Input: part model. Units: mm. Frame: model coordinates. A direction names the side the tool comes from. Round coordinates to 2 decimals unless told otherwise and drop trailing zeros. Loops run counter-clockwise (first coordinate to the right, second up) from the corner with the lowest first, then second, coordinate; pieces in that order, holes last.
(1) Access query for faces 5 (the face through (-0.8, -9.6, 200)), 6 (the face through (-0.521, 9.507, -138.034)), 7 (the face through (9, 0, 3)). Directions: +Z, -Z, +X, -X, +Y, -Y. A direction counts if a zero-diameter tool reaches every point of the face in a straight line with its end or side. Return the directions, or none.
(2) Cut plane A-A, the plane z = -79. Output: boundary loops of the cut face in (x, y).
(3) Line query: line 1 (Y direction, x = 7, z = -19); line 2 (X direction, y = 9.75, z = 189.5) (3 decimals). Output: solid intervals per line, ascending.
(4) Draft query along Z for faces 1 (the face through (0, 9, 3)), 2 (the face through (-0.8, -9.6, -200)), 3 (the face through (-0.521, 9.507, -123.034)), 4 (the face through (-0.521, 9.507, 123.034)). Return one class per face: released by +Z, released by -Z, zero draft, split by the parting line, or undercut.
(5) Cut plane B-B, the plane y = -2.75. Output: boundary loops of the cut face in (x, z).
(6) First-contact query: pin 1 Ø3.5 at (x, z) = (0, -189.5) entering from -Y; pin 2 Ø6.5 at (x, z) = (0, -142) entering from +Y. Flat tips, straight axial feed; report the tip coordinate or a pass-through.
from build123d import *

# Parameters (mm, degrees)
SKETCH_1_W               = 20
SKETCH_1_H               = 20
EXTRUDE_1_DEPTH          = 200
SKETCH_2_W               = 18
SKETCH_2_H               = 18
CUT_EXTRUDE_1_DEPTH      = 201
CUT_EXTRUDE_1_DEPTH_BACK = 201
CUT_EXTRUDE_START        = -21
SKETCH_3_R               = 1.525
CUT_EXTRUDE_2_DEPTH      = 22
SKETCH_4_R               = 1.525
CUT_EXTRUDE_3_DEPTH      = 22
SKETCH_5_R               = 2.025
CUT_EXTRUDE_4_DEPTH      = 22
SKETCH_8_R               = 4
CUT_EXTRUDE_5_DEPTH      = 3


with BuildPart() as part:
    # 草图1 → 凸台-拉伸1 (new body, symmetric)
    with BuildSketch(Plane.XY):
        Rectangle(SKETCH_1_W, SKETCH_1_H)
    extrude(amount=EXTRUDE_1_DEPTH, both=True)

    # 草图2 → 切除-拉伸1 (cut, two sides)
    with BuildSketch(Plane.XY) as cut_extrude_1_sk:
        Rectangle(SKETCH_2_W, SKETCH_2_H)
    extrude(amount=CUT_EXTRUDE_1_DEPTH, mode=Mode.SUBTRACT)
    extrude(cut_extrude_1_sk.sketch, amount=-CUT_EXTRUDE_1_DEPTH_BACK, mode=Mode.SUBTRACT)

    # 草图3 → 切除-拉伸2 (cut)
    with BuildSketch(Plane(origin=(0, 10, 0), x_dir=(1, 0, 0), z_dir=(0, 1, 0)).offset(CUT_EXTRUDE_START)):
        with Locations((0, -189.5)):
            Circle(SKETCH_3_R)
        with Locations((0, -169.5)):
            Circle(SKETCH_3_R)
    cut_extrude_2 = extrude(amount=CUT_EXTRUDE_2_DEPTH, mode=Mode.SUBTRACT)

    # 镜向1: 切除-拉伸2 across plane
    add(cut_extrude_2.mirror(Plane.XY), mode=Mode.SUBTRACT)

    # 草图4 → 切除-拉伸3 (cut)
    with BuildSketch(Plane(origin=(10, 0, 0), x_dir=(0, 0, -1), z_dir=(1, 0, 0)).offset(CUT_EXTRUDE_START)):
        with Locations((-179.5, 6)):
            Circle(SKETCH_4_R)
        with Locations((-159.5, 6)):
            Circle(SKETCH_4_R)
    cut_extrude_3 = extrude(amount=CUT_EXTRUDE_3_DEPTH, mode=Mode.SUBTRACT)

    # 草图5 → 切除-拉伸4 (cut)
    with BuildSketch(Plane.XZ.offset(10).offset(CUT_EXTRUDE_START)):
        with Locations((0, 142)):
            Circle(SKETCH_5_R)
        with Locations((0, 127)):
            Circle(SKETCH_5_R)
    cut_extrude_4 = extrude(amount=CUT_EXTRUDE_4_DEPTH, mode=Mode.SUBTRACT)

    # 草图8 → 切除-拉伸5 (cut)
    with BuildSketch(Plane(origin=(0, 10, 0), x_dir=(1, 0, 0), z_dir=(0, 1, 0))):
        with Locations((0, -127)):
            Circle(SKETCH_8_R)
        with Locations((0, -142)):
            Circle(SKETCH_8_R)
    cut_extrude_5 = extrude(amount=-CUT_EXTRUDE_5_DEPTH, mode=Mode.SUBTRACT)

    # 镜向2: 切除-拉伸4, 切除-拉伸5 across plane
    add(cut_extrude_4.mirror(Plane.XY), mode=Mode.SUBTRACT)
    add(cut_extrude_5.mirror(Plane.XY), mode=Mode.SUBTRACT)

    # 镜向3: 切除-拉伸3 across plane
    add(cut_extrude_3.mirror(Plane.XY), mode=Mode.SUBTRACT)


solid = part.part
Reported:
1. face 5: +Z, +X, -X, +Y, -Y
1. face 6: +Y
1. face 7: +Z, -Z
2. outline: (-10, -10) - (10, -10) - (10, 10) - (-10, 10) - close; hole (-9, -9) - (9, -9) - (9, 9) - (-9, 9) - close
3. line 1: y = -10 to -9, 9 to 10
3. line 2: x = -10 to -1.525, 1.525 to 10
4. face 1: zero draft
4. face 2: released by -Z
4. face 3: undercut
4. face 4: undercut
5. outline: (-10, -200) - (-9, -200) - (-9, 200) - (-10, 200) - close; (9, -200) - (10, -200) - (10, 200) - (9, 200) - close
6. pin 1: stops at y = -10
6. pin 2: stops at y = -9
